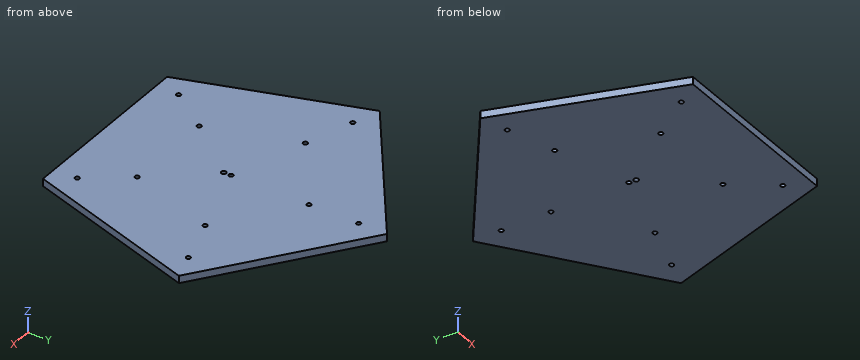
```python
from build123d import *

# Parameters (mm, degrees)
BOSS_EXTRUDE1_DEPTH = 3
SKETCH3_R           = 0.9
CUT_EXTRUDE1_DEPTH  = 3
SKETCH5_R           = 0.9
CUT_EXTRUDE2_DEPTH  = 3
CIRPATTERN1_COUNT   = 5
SKETCH6_R           = 1
CUT_EXTRUDE3_DEPTH  = 3


with BuildPart() as part:
    # Sketch1 → Boss-Extrude1 (new body)
    with BuildSketch(Plane.XY):
        Polygon((-37.706506674, -51.464286136), (37.293493326, -51.764357899), (60.755153109, 19.472153549), (0.255256287, 63.798810626), (-60.597396047, 19.95767986), align=None)
    extrude(amount=BOSS_EXTRUDE1_DEPTH)

    # Sketch3 → Cut-Extrude1 (cut)
    with BuildSketch(Plane.XY.offset(3)):
        Circle(SKETCH3_R)
    extrude(amount=-CUT_EXTRUDE1_DEPTH, mode=Mode.SUBTRACT)

    # Sketch5 → Cut-Extrude2 (cut)
    with BuildSketch(Plane.XY.offset(3)):
        with Locations((-30.864859889, -42.126362822)):
            Circle(SKETCH5_R)
        with Locations((-18.84066677, -25.714964105)):
            Circle(SKETCH5_R)
    cut_extrude2 = extrude(amount=-CUT_EXTRUDE2_DEPTH, mode=Mode.SUBTRACT)

    # CirPattern1: Cut-Extrude2 ×5 about axis
    cirpattern1_axis = Axis((0, 0, 0), (0, 0, 1))
    for i in range(1, CIRPATTERN1_COUNT):
        add(cut_extrude2.rotate(cirpattern1_axis, i * 360 / CIRPATTERN1_COUNT), mode=Mode.SUBTRACT)

    # Sketch6 → Cut-Extrude3 (cut)
    with BuildSketch(Plane(origin=(0, 0, 0), x_dir=(-1, 0, 0), z_dir=(0, 0, -1))):
        with Locations((0, -3)):
            Circle(SKETCH6_R)
    extrude(amount=-CUT_EXTRUDE3_DEPTH, mode=Mode.SUBTRACT)


solid = part.part
```
Model file for the job. Use its own axes, mm. Coordinates: 2 decimals unless noted, no trailing zeros. Order: outer loops, then holes, each group sorted by start corner. A loop starts at its lowest first (then second) coordinate and runs counter-clockwise, first axis right, second up. Notation, with made-up numbers: (-12, -5.5) -> (36, -5.5) arc R7 ccw to (36, -1.5) -> close; hole circle Ø6 at (-26.75, 12). An arc over 180 degrees is marked (long way). Answer as a JSON object with one key per item and string values. Group by question number.
1) Cut at C-C, the plane y = 24.5. Write the cut outline in (x, z), then the cut area to 3 significant figures.
2) Cut at B-B, the plane x = 35. Write the cut outline in (y, z), then the cut area to 3 significant figures.
3) Drill centre lines: L1, parallel to Y at x = 0, z = 2.25; L2, parallel to X at y = -42.5, z = 1.35; L3, parallel to X at y = -13, z = 0.2. Where is each one in solid material? Low to high.
4) Flat gauge pins, fed straight in: pin 1 (1.5 mm diameter, centred on y = -38.5, z = 2.5, fed in from +X); pin 2 (1.5 mm diameter, centred on x = -13, z = 1, fed in from -Y). Where does each tip first touch, or does it go through?
5) Cut at A-A, the plane z = 0.9. Count the separate pieces of the cut face and the enclosed holes in it, then the cut area to 3 significant figures.
Check values:
{
 "1": {"outline": "(-54.29, 0) -> (53.89, 0) -> (53.89, 3) -> (-54.29, 3) -> close", "area": "325 mm²"},
 "2": {"outline": "(-51.76, 0) -> (38.34, 0) -> (38.34, 3) -> (-51.76, 3) -> close", "area": "270 mm²"},
 "3": {"L1": "y = -51.62 to -4, -2 to -0.9, 0.9 to 30.99, 32.77 to 51.35, 53.1 to 63.61", "L2": "x = -40.58 to -31.68, -30.05 to 29.64, 31.42 to 40.34", "L3": "x = -50.03 to 50.06"},
 "4": {"pin 1": "stops at x = 41.91", "pin 2": "stops at y = -51.57"},
 "5": {"separate pieces": "1", "enclosed holes": "12", "area": "9,650 mm²"}
}
